from build123d import *

# Parameters (mm, degrees)
F1_DEPTH = 25.4
F2_W     = 25.8318
F2_H     = 12.7
F3_DEPTH = 25.4
F5_DEPTH = 25.4
F6_W     = 6.35
F6_H     = 12.7
F7_DEPTH = 25.4
F8_R     = 6.35
F9_DEPTH = 25.4


with BuildPart() as f1:
    # F0 (on Front) → F1 (new body)
    with BuildSketch(Plane.XZ):
        Polygon((0, 25.4), (0, 0), (38.1, 0), (38.1, 25.4), (12.7, 25.4), align=None)
    extrude(amount=F1_DEPTH)

    # F2 (on face) → F3 (cut)
    with BuildSketch(Plane.XY.offset(25.4)):
        with Locations((25.1841, -19.05)):
            Rectangle(F2_W, F2_H)
    extrude(amount=-F3_DEPTH, mode=Mode.SUBTRACT)

    # F4 (on face) → F5 (cut)
    with BuildSketch(Plane.XZ.offset(12.7)):
        with BuildLine():
            Line((38.1, 25.4), (25.1841, 25.4))
            ThreePointArc((25.1841, 25.4), (37.8841, 12.7), (25.1841, 0))
            Line((25.1841, 0), (38.1, 0))
            Line((38.1, 0), (38.1, 25.4))
        make_face()
    extrude(amount=-F5_DEPTH, mode=Mode.SUBTRACT)

    # F6 (on face) → F7 (cut)
    with BuildSketch(Plane.YZ.offset(12.2682)):
        with Locations((-22.225, 12.7)):
            Rectangle(F6_W, F6_H)
    extrude(amount=-F7_DEPTH, mode=Mode.SUBTRACT)

    # F8 (on face) → F9 (cut)
    with BuildSketch(Plane.XZ.offset(12.7)):
        with Locations((25.1841, 12.7)):
            Circle(F8_R)
    extrude(amount=-F9_DEPTH, mode=Mode.SUBTRACT)


solid = f1.part
Part model, mm, in its own coordinate system. A direction names the side the tool comes from. Coordinates: 2 decimals unless noted, no trailing zeros. Write each loop counter-clockwise with the first axis right and the second up, starting at its lowest first coordinate (ties: lowest second). Pieces come first, ordered by that corner, then holes. Notation, with made-up numbers: M 17.25,32 L 24.25,32 A24 cw 24.25,46 Z; hole C 13,47 d11. An arc over 180 degrees is marked long. Return JSON: item names as keys, results as strings.
1. 3-axis set-ups, long thin cutter, end or side, ignore diameter. For faces 1 (the face through (10, -10, 0)), 2 (the face through (12.268, -18, 13)), 3 (the face through (6, -22, 6.35)): which of +Z, -Z, +X, -X, +Y, -Y reach the whole face in a straight line?
Determined:
{"face 1": "-Z, +X, -X, +Y, -Y", "face 2": "+Z, -Z, +X, -Y", "face 3": "+X, -X, -Y"}
2. Saw through at B-B, the plane y = -20.5. Write the cut outline in (x, z).
Determined:
{"outline": "M 0,0 L 12.27,0 L 12.27,6.35 L 0,6.35 Z; M 0,19.05 L 12.27,19.05 L 12.27,25.4 L 0,25.4 Z"}
3. Saw through at D-D, the plane y = -7.5. Write the cut outline in (x, z).
Determined:
{"outline": "M 0,0 L 25.18,0 A12.7 ccw 25.18,25.4 L 0,25.4 Z; hole C 25.18,12.7 d12.7"}
4. Probe L1, parallel to Z at x = 3, y = -21.75; L2, parallel to X at y = -14.75, z = 11.5; L3, parallel to Y at x = 32, z = 14. List the from-to ranges inside material, lowest first.
Determined:
{"L1": "0 to 6.35, 19.05 to 25.4", "L2": "0 to 12.27", "L3": "-12.7 to 0"}
5. Flat gauge pins, fed straight in: pin 1 Ø4 at (x, z) = (12.5, 10) entering from -Y; pin 2 Ø1 at (x, y) = (31.5, -9) entering from +Z; pin 3 Ø4 at (y, z) = (-20, 9) entering from +X. Where does each tip first touch, or does it go through?
Determined:
{"pin 1": "y = -19.05", "pin 2": "z = 23.99", "pin 3": "x = 12.27"}
6. Saw through at C-C, the plane x = 4. Write the cut outline in (y, z), then the cut area to 3 significant figures.
Determined:
{"outline": "M -25.4,0 L 0,0 L 0,25.4 L -25.4,25.4 L -25.4,19.05 L -19.05,19.05 L -19.05,6.35 L -25.4,6.35 Z", "area": "565 mm²"}
7. Saw through at A-A, the plane z = 12.7. Write the cut outline in (x, y).
Determined:
{"outline": "M 0,-19.05 L 12.27,-19.05 L 12.27,-12.7 L 18.83,-12.7 L 18.83,0 L 0,0 Z; M 31.53,-12.7 L 37.88,-12.7 L 37.88,0 L 31.53,0 Z"}
